Verification items for the finished model (mm, model axes). A direction names the side the tool comes from. Give positions to 0.01 mm unless a question says otherwise; leave off trailing zeros. Loops run counter-clockwise (first coordinate to the right, second up) from the corner with the lowest first, then second, coordinate; pieces in that order, holes last. Notation, with made-up numbers: (89.25, 60.5) - (145.25, 60.5) arc R14 ccw to (145.25, 75.5) - close; hole circle Ø8 at (15.5, 87). An arc over 180 degrees is marked (long way). Use one line per item in the form item = value.
```python
from build123d import *

# Parameters (mm, degrees)
F0_W     = 35.56
F0_H     = 35.56
F0_W_2   = 15.875
F0_H_2   = 15.875
F1_DEPTH = 1.27
F2_R     = 2.54
F3_R     = 1.27


with BuildPart() as f1:
    # F0 (on Top) → F1 (new body)
    with BuildSketch(Plane.XY):
        Rectangle(F0_W, F0_H)
        with Locations((-8.5725, -8.5725)):
            Rectangle(F0_W_2, F0_H_2, mode=Mode.SUBTRACT)
        with Locations((8.5725, -8.5725)):
            Rectangle(F0_W_2, F0_H_2, mode=Mode.SUBTRACT)
        with Locations((-8.5725, 8.5725)):
            Rectangle(F0_W_2, F0_H_2, mode=Mode.SUBTRACT)
        with Locations((8.5725, 8.5725)):
            Rectangle(F0_W_2, F0_H_2, mode=Mode.SUBTRACT)
    extrude(amount=-F1_DEPTH)

    # F2
    f2_edges = [f1.edges().sort_by_distance(p)[0] for p in [
        (-17.78, -17.78, -0.635),
        (17.78, -17.78, -0.635),
        (17.78, 17.78, -0.635),
        (-17.78, 17.78, -0.635),
    ]]
    fillet(f2_edges, radius=F2_R)

    # F3
    f3_edges = [f1.edges().sort_by_distance(p)[0] for p in [
        (-16.51, 16.51, -0.635),
        (16.51, 16.51, -0.635),
        (16.51, -16.51, -0.635),
        (-16.51, -16.51, -0.635),
    ]]
    fillet(f3_edges, radius=F3_R)


solid = f1.part
```
1. Draft check along X on faces 3 (the flat face through (17.78, 0, -1)), 4 (the cylindrical face through (-17.056, -17.016, -0.644)), 5 (the flat face through (-9, 0.635, -1)). Enter one of: released by +X, released by -X, zero draft, split by the parting line, or undercut.
Result set:
face_3 = released by +X
face_4 = released by -X
face_5 = undercut
2. Section check C-C, the plane z = -1.05. Record the cut outline in (x, y) (3 decimals), then the cut area to 3 significant figures.
Result set:
outline = (-17.78, -15.24) arc R2.54 ccw to (-15.24, -17.78) - (15.24, -17.78) arc R2.54 ccw to (17.78, -15.24) - (17.78, 15.24) arc R2.54 ccw to (15.24, 17.78) - (-15.24, 17.78) arc R2.54 ccw to (-17.78, 15.24) - close; hole (-16.51, -15.24) arc R1.27 ccw to (-15.24, -16.51) - (-0.635, -16.51) - (-0.635, -0.635) - (-16.51, -0.635) - close; hole (-16.51, 0.635) - (-0.635, 0.635) - (-0.635, 16.51) - (-15.24, 16.51) arc R1.27 ccw to (-16.51, 15.24) - close; hole (0.635, -16.51) - (15.24, -16.51) arc R1.27 ccw to (16.51, -15.24) - (16.51, -0.635) - (0.635, -0.635) - close; hole (0.635, 0.635) - (16.51, 0.635) - (16.51, 15.24) arc R1.27 ccw to (15.24, 16.51) - (0.635, 16.51) - close
area = 252 mm²
3. Scan lines: probe 1 along Y at (x, z) = (-6, -1.2) (3 decimals); probe 2 along X at (y, z) = (16, -1.1) (1 decimal). Record each from-to range of solid material in increasing order.
Result set:
probe_1 = -17.78 to -16.51, -0.635 to 0.635, 16.51 to 17.78
probe_2 = -17.7 to -16.3, -0.6 to 0.6, 16.3 to 17.7
4. Section check A-A, the plane y = 8.5. Record the cut outline in (x, z) (3 decimals).
Result set:
outline = (-17.78, -1.27) - (-16.51, -1.27) - (-16.51, 0) - (-17.78, 0) - close; (-0.635, -1.27) - (0.635, -1.27) - (0.635, 0) - (-0.635, 0) - close; (16.51, -1.27) - (17.78, -1.27) - (17.78, 0) - (16.51, 0) - close
5. Tool access check on faces 1 (the cylindrical face through (-16.128, -16.148, -0.644)), 2 (the cylindrical face through (-17.056, 17.016, -0.644)). Record the directions out of +Z, -Z, +X, -X, +Y, -Y that give a thin tool (end or side, any length) a straight path to the whole face; none if there is none.
Result set:
face_1 = +Z, -Z
face_2 = +Z, -Z, -X, +Y
